Can you work these out from the drawing? Everything is in mm from the part's minimum corner. A direction names the side the tool comes from. Round coordinates to 2 decimals unless told otherwise and drop trailing zeros. Order: outer loops, then holes, each group sorted by start corner. A loop starts at its lowest first (then second) coordinate and runs counter-clockwise, first axis right, second up. Notation, with made-up numbers: (46.5, 63.5) - (59.5, 63.5) arc R34 ccw to (59.5, 100.5) - close; hole circle Ø4 at (19, 41). An arc over 180 degrees is marked (long way). Answer as a JSON object with one key per item and string values.
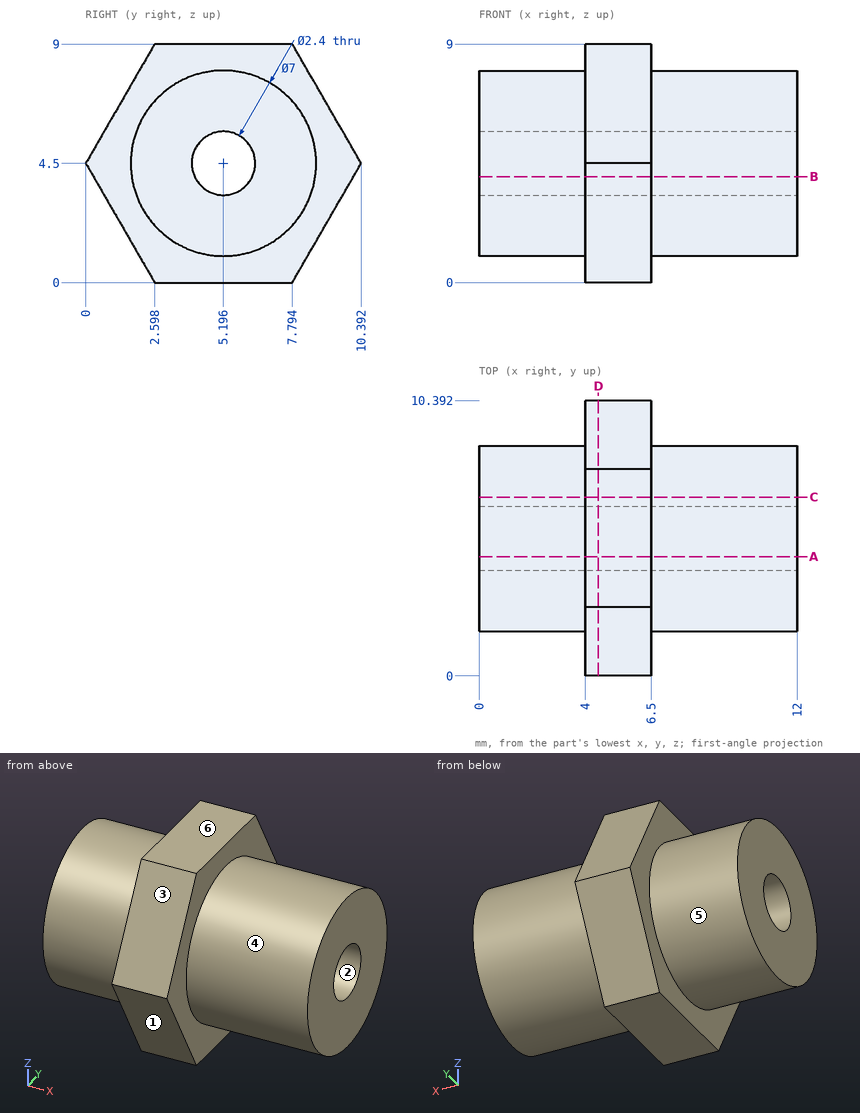
1. Imagine slicing it at D-D (x = 4.5). List the corners of the cut face in (y, z) for me.
Responses:
{"outline": "(0, 4.5) - (2.6, 0) - (7.79, 0) - (10.39, 4.5) - (7.79, 9) - (2.6, 9) - close; hole circle Ø2.4 at (5.2, 4.5)"}
2. For the marked faces 4, 5 and 6, which set-ups out of +Z, -Z, +X, -X, +Y, -Y let a thin tool reach every point of the face, with its end or its side?
Responses:
{"face 4": "+X", "face 5": "-X", "face 6": "+Z, +X, -X, +Y, -Y"}
3. Imagine slicing it at A-A (y = 4.5). List the corners of the cut face in (x, z) for me.
Responses:
{"outline": "(0, 1.07) - (4, 1.07) - (4, 0) - (6.5, 0) - (6.5, 1.07) - (12, 1.07) - (12, 3.52) - (0, 3.52) - close; (0, 5.48) - (12, 5.48) - (12, 7.93) - (6.5, 7.93) - (6.5, 9) - (4, 9) - (4, 7.93) - (0, 7.93) - close"}
4. Thinking about a two-plate mould opening in Z: for the marked faces 1, 2 and 3, which applies, pulls with the +Z half, pulls with the -Z half, needs draft (parallel to the pull), parting line crosses it, or undercut?
Responses:
{"face 1": "pulls with the -Z half", "face 2": "undercut", "face 3": "pulls with the +Z half"}
5. Imagine slicing it at C-C (y = 6.75). List the corners of the cut face in (x, z) for me, plus the area to 3 significant figures.
Responses:
{"outline": "(0, 1.36) - (4, 1.36) - (4, 0) - (6.5, 0) - (6.5, 1.36) - (12, 1.36) - (12, 7.64) - (6.5, 7.64) - (6.5, 9) - (4, 9) - (4, 7.64) - (0, 7.64) - close", "area": "82.1 mm2"}
6. For P1, Ø1.5, axis at x = 9.5, z = 4.5, coming from the -Y side; P2, Ø3, axis at x = 7, z = 6.5, coming from the -Y side; P3, Ø5, axis at x = 1, y = 7.5, coming from the +Z side, each with a flat end and sliding along its axis, tell me the tip position at first contact or that it passes through.
Responses:
{"P1": "y = 1.7", "P2": "y = 0.34", "P3": "z = 8"}
7. Imagine slicing it at B-B (z = 4). List the corners of the cut face in (x, y) for me (1 decimal).
Responses:
{"outline": "(0, 1.7) - (4, 1.7) - (4, 0.3) - (6.5, 0.3) - (6.5, 1.7) - (12, 1.7) - (12, 4.1) - (0, 4.1) - close; (0, 6.3) - (12, 6.3) - (12, 8.7) - (6.5, 8.7) - (6.5, 10.1) - (4, 10.1) - (4, 8.7) - (0, 8.7) - close"}
8. If I drill on L1, parallel to X at y = 7.5, z = 1; L2, parallel to Y at x = 8, z = 4.5; L3, parallel to Z at x = 3.5, y = 3.25, over which ranges is the centre line in solid material (lowest first)? Write a range as [from, to].
Responses:
{"L1": "[4, 6.5]", "L2": "[1.7, 4], [6.4, 8.7]", "L3": "[1.59, 7.41]"}
